The listing builds one solid part. Answer for the finished solid, in the listing's coordinates (mm). Coordinates: 2 decimals unless noted, no trailing zeros. Order: outer loops, then holes, each group sorted by start corner. A loop starts at its lowest first (then second) coordinate and runs counter-clockwise, first axis right, second up.
from build123d import *

# Parameters (mm, degrees)
SKETCH1_R           = 3.175
SKETCH1_R_2         = 4.7625
BOSS_EXTRUDE1_DEPTH = 6.35


with BuildPart() as part:
    # Sketch1 → Boss-Extrude1 (new body)
    with BuildSketch(Plane(origin=(0, 0, 0), x_dir=(0, 0, -1), z_dir=(1, 0, 0))):
        with BuildLine():
            Line((12.7, 50.8), (12.7, -50.8))
            ThreePointArc((12.7, -50.8), (0, -63.5), (-12.7, -50.8))
            Line((-12.7, -50.8), (-12.7, 50.8))
            ThreePointArc((-12.7, 50.8), (0, 63.5), (12.7, 50.8))
        make_face()
        with Locations((0, 50.8)):
            Circle(SKETCH1_R, mode=Mode.SUBTRACT)
        Circle(SKETCH1_R, mode=Mode.SUBTRACT)
        with Locations((0, -50.8)):
            Circle(SKETCH1_R_2, mode=Mode.SUBTRACT)
    extrude(amount=BOSS_EXTRUDE1_DEPTH)


solid = part.part
(1) Find the intervals of material crossed by probe 1 along Y at (x, z) = (4.5, 0) (1 decimal); probe 2 along Y at (x, z) = (4.75, 2.75); probe 3 along Y at (x, z) = (4, 5.5), in increasing order.
(2) Given pin 1 Ø2 at (x, z) = (3, -6) entering from -Y, flat-ended and moving along its own axis, determine where the tip first touches the part or whether it passes through.
(3) Find section A-A on y = 0. Determine the outline of the cut face in (x, z) (3 decimals), then the cut area to 3 significant figures.
(4) The mould has two halves that part along Z. Classify faces 1 (the cylindrical face through (3.131, 63.497, 0.279)), 2 (the cylindrical face through (3.13, -3.1, 0.69)), 3 (the flat face through (3, -1, 12.7)): pulls with the +Z half, pulls with the -Z half, needs draft (parallel to the pull), parting line crosses it, or undercut.
(5) Find section B-B on z = 0.25. Determine the outline of the cut face in (x, y), then the cut area to 3 significant figures.
(6) Find section D-D on z = -7.25. Determine the outline of the cut face in (x, y).
(7) Find section C-C on x = 1.75. Count the separate pieces of the cut face and the enclosed holes in it, then the cut area to 3 significant figures.
Resolved:
1. probe 1: y = -63.5 to -55.6, -46 to -3.2, 3.2 to 47.6, 54 to 63.5
1. probe 2: y = -63.2 to -54.69, -46.91 to -1.59, 1.59 to 49.21, 52.39 to 63.2
1. probe 3: y = -62.25 to 62.25
2. pin 1: stops at y = -62.47
3. outline: (0, -12.7) - (6.35, -12.7) - (6.35, -3.175) - (0, -3.175) - close; (0, 3.175) - (6.35, 3.175) - (6.35, 12.7) - (0, 12.7) - close
3. area: 121 mm2
4. face 1: parting line crosses it
4. face 2: undercut
4. face 3: pulls with the +Z half
5. outline: (0, -63.5) - (6.35, -63.5) - (6.35, -55.56) - (0, -55.56) - close; (0, -46.04) - (6.35, -46.04) - (6.35, -3.17) - (0, -3.17) - close; (0, 3.17) - (6.35, 3.17) - (6.35, 47.63) - (0, 47.63) - close; (0, 53.97) - (6.35, 53.97) - (6.35, 63.5) - (0, 63.5) - close
5. area: 666 mm2
6. outline: (0, -61.23) - (6.35, -61.23) - (6.35, 61.23) - (0, 61.23) - close
7. separate pieces: 1
7. enclosed holes: 3
7. area: 2,950 mm2
